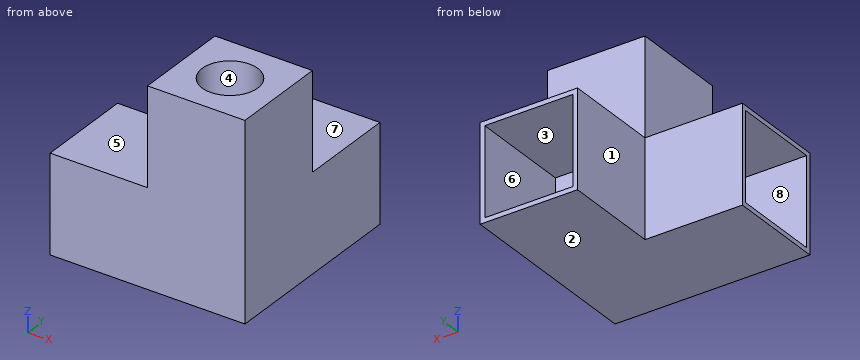
from build123d import *

# Parameters (mm, degrees)
F0_W      = 42
F0_H      = 42
F1_DEPTH  = 42
F2_W      = 21
F2_H      = 21
F3_DEPTH  = 42
F4_W      = 21
F4_H      = 21
F5_DEPTH  = 21
F6_W      = 21
F6_H      = 21
F7_DEPTH  = 21
F9_W      = 19
F9_H      = 19
F10_DEPTH = 41
F11_W     = 19
F11_H     = 19
F12_DEPTH = 22
F8_R      = 6
F13_DEPTH = 18
F15_DEPTH = 19


with BuildPart() as f1:
    # F0 (on Top) → F1 (new body)
    with BuildSketch(Plane.XY):
        Rectangle(F0_W, F0_H)
    extrude(amount=F1_DEPTH)

    # F2 (on face) → F3 (cut, through all)
    with BuildSketch(Plane.XY.offset(42)):
        with Locations((-10.5, 10.5)):
            Rectangle(F2_W, F2_H)
    extrude(amount=-F3_DEPTH, mode=Mode.SUBTRACT)

    # F4 (on face) → F5 (cut, through all)
    with BuildSketch(Plane.XZ.offset(21)):
        with Locations((-10.5, 31.5)):
            Rectangle(F4_W, F4_H)
    extrude(amount=-F5_DEPTH, mode=Mode.SUBTRACT)

    # F6 (on face) → F7 (cut, through all)
    with BuildSketch(Plane.YZ.offset(21)):
        with Locations((10.5, 31.5)):
            Rectangle(F6_W, F6_H)
    extrude(amount=-F7_DEPTH, mode=Mode.SUBTRACT)

    # F9 (on face) → F10 (cut)
    with BuildSketch(Plane(origin=(-21, 0, 0), x_dir=(0, -1, 0), z_dir=(-1, 0, 0))):
        with Locations((10.5, 10.5)):
            Rectangle(F9_W, F9_H)
    extrude(amount=-F10_DEPTH, mode=Mode.SUBTRACT)

    # F11 (on face) → F12 (cut)
    with BuildSketch(Plane(origin=(0, 21, 0), x_dir=(-1, 0, 0), z_dir=(0, 1, 0))):
        with Locations((-10.5, 10.5)):
            Rectangle(F11_W, F11_H)
    extrude(amount=-F12_DEPTH, mode=Mode.SUBTRACT)

    # F8 (on face) → F13 (cut)
    with BuildSketch(Plane.XY.offset(42)):
        with Locations((10.5, -10.5)):
            Circle(F8_R)
    extrude(amount=-F13_DEPTH, mode=Mode.SUBTRACT)

    # F14 (on face) → F15 (join, through all)
    with BuildSketch(Plane.XY.offset(1)):
        Polygon((20, -1), (6, -1), (6, -6), (1, -6), (1, -20), (20, -20), align=None)
    extrude(amount=F15_DEPTH)


solid = f1.part
Geometry check sheet. Reference: the model listing, model coordinates, mm. Face numbers are marked on the shaded views. A direction names the side the tool comes from. Round coordinates to 2 decimals unless told otherwise and drop trailing zeros. Loops run counter-clockwise (first coordinate to the right, second up) from the corner with the lowest first, then second, coordinate; pieces in that order, holes last.
Item 1: Cross-section at A-A on z = 12.5. Record the boundary of the cut face in (x, y), then the cut area to 3 significant figures.
Item 2: Cross-section at D-D on x = 10.5. Record the boundary of the cut face in (y, z), then the cut area to 3 significant figures.
Item 3: Access from +Z, -Z, +X, -X, +Y, -Y to the whole of each face (thin tool, end or side, straight path). Record for the marked faces 5, 6, 7 and 8.
Item 4: Cross-section at B-B on x = -11. Record the boundary of the cut face in (y, z), then the cut area to 3 significant figures.
Item 5: Cross-section at C-C on y = 13. Record the boundary of the cut face in (x, z), then the cut area to 3 significant figures.
Item 6: Mould release check, pull along X, two halves, no side actions. Record for the marked faces 1, 2, 3 and 4: pulls with the +X half, pulls with the -X half, needs draft (parallel to the pull), parting line crosses it, or undercut.
Item 7: Gauge pin test, flat ends, axial feed: pin 1 (7 mm diameter, centred on x = 12.5, z = 13, fed in from +Y); pin 2 (6.5 mm diameter, centred on x = 9, z = 34, fed in from +Y); pin 3 (1.5 mm diameter, centred on y = -4, z = 9.5, fed in from -X); pin 4 (11 mm diameter, centred on x = 10.5, y = -10.5, fed in from -Z). Record the tip position at first contact, or that the pin passes through.
Item 8: Thickness scan on line 1 (Z direction, x = 16.5, y = 8); line 2 (Y direction, x = 10.5, z = 28); line 3 (X direction, y = -2, z = 34). Record the ranges inside material, lowest first.
Answer sheet:
1. outline: (-21, -21) - (21, -21) - (21, 21) - (20, 21) - (20, -1) - (6, -1) - (6, -6) - (1, -6) - (1, -20) - (-21, -20) - close; (-21, -1) - (1, -1) - (1, 21) - (0, 21) - (0, 0) - (-21, 0) - close
1. area: 462 mm2
2. outline: (-21, 0) - (21, 0) - (21, 1) - (-1, 1) - (-1, 20) - (21, 20) - (21, 21) - (0, 21) - (0, 42) - (-4.5, 42) - (-4.5, 24) - (-16.5, 24) - (-16.5, 42) - (-21, 42) - close
2. area: 689 mm2
3. face 5: +Z, -X, +Y, -Y
3. face 6: +Y
3. face 7: +Z, +X, -X, +Y
3. face 8: -X
4. outline: (-21, 0) - (0, 0) - (0, 21) - (-21, 21) - close; hole (-20, 1) - (-1, 1) - (-1, 20) - (-20, 20) - close
4. area: 80.0 mm2
5. outline: (0, 0) - (21, 0) - (21, 21) - (0, 21) - close; hole (1, 1) - (20, 1) - (20, 20) - (1, 20) - close
5. area: 80.0 mm2
6. face 1: pulls with the -X half
6. face 2: needs draft
6. face 3: undercut
6. face 4: undercut
7. pin 1: stops at y = -1
7. pin 2: stops at y = 0
7. pin 3: stops at x = 6
7. pin 4: stops at z = 0
8. line 1: z = 0 to 1, 20 to 21
8. line 2: y = -21 to -16.5, -4.5 to 0
8. line 3: x = 0 to 21
